For this review, take the finished solid that the model builds, in its own axes (mm). A direction names the side the tool comes from. Give positions to 0.01 mm unless a question says otherwise; leave off trailing zeros. Write each loop counter-clockwise with the first axis right and the second up, starting at its lowest first coordinate (ties: lowest second). Pieces come first, ordered by that corner, then holes. Notation, with made-up numbers: (-4.75, 9.5) -> (3.25, 9.5) arc R9 cw to (3.25, 24.5) -> close; hole circle Ø9 at (28, 30). An arc over 180 degrees is marked (long way). Write item = value, one per line.
```python
from build123d import *

# Parameters (mm, degrees)
CIRPATTERN1_COUNT         = 12
F_8_CLEARANCE_HOLE1_D     = 4.4958
F_8_CLEARANCE_HOLE1_DEPTH = 9.652
F_8_CLEARANCE_HOLE1_TIP   = 1.350674586


with BuildPart() as part:
    # Sketch1 → Revolve1 (revolve)
    with BuildSketch(Plane.XY, mode=Mode.PRIVATE) as revolve1_sk:
        Polygon((0, 0), (-30.6832, 0), (-30.6832, -7.8994), (-29.7942, -7.8994), (-29.7942, -12.319), (-26.1112, -12.319), (-26.1112, -6.223), (0, -6.223), align=None)
    revolve(revolve1_sk.sketch.rotate(Axis((0, -6.223, 0), (0, 1, 0)), 270), axis=Axis((0, -6.223, 0), (0, 1, 0)))

    # Sketch3 → D (0.246) Diameter Hole1 (revolve, cut)
    with BuildSketch(Plane(origin=(0, 0, -21.59), x_dir=(0, 0, 1), z_dir=(1, 0, 0))):
        Polygon((0, 0), (0, 14.577208746), (3.1242, 12.7), (3.1242, 0), align=None)
    d_0_246_diameter_hole1 = revolve(axis=Axis((0, 6.35, -21.59), (0, -1, 0)), mode=Mode.SUBTRACT)

    # CirPattern1: D (0.246) Diameter Hole1 ×12 about axis
    cirpattern1_axis = Axis((0, 0, 0), (0, 1, 0))
    for i in range(1, CIRPATTERN1_COUNT):
        add(d_0_246_diameter_hole1.rotate(cirpattern1_axis, i * 360 / CIRPATTERN1_COUNT), mode=Mode.SUBTRACT)

    # #8 Clearance Hole1
    with Locations(Plane.XZ.offset(6.223)):
        with Locations((0, 0)):
            Hole(F_8_CLEARANCE_HOLE1_D / 2, depth=F_8_CLEARANCE_HOLE1_DEPTH)
            with Locations((0, 0, -(F_8_CLEARANCE_HOLE1_DEPTH + F_8_CLEARANCE_HOLE1_TIP / 2))):  # 118° drill point
                Cone(0, F_8_CLEARANCE_HOLE1_D / 2, F_8_CLEARANCE_HOLE1_TIP, mode=Mode.SUBTRACT)


solid = part.part
```
(1) Take a section at C-C (z = -10.5). Write out the cut boundary in (x, y), plus the area to 3 significant figures.
Answers below:
outline = (-28.83, -7.9) -> (-27.88, -7.9) -> (-27.88, -12.32) -> (-23.91, -12.32) -> (-23.91, -6.22) -> (-21.81, -6.22) -> (-21.81, 0) -> (-28.83, 0) -> close; (-15.59, -6.22) -> (15.59, -6.22) -> (15.59, 0) -> (-15.59, 0) -> close; (21.81, -6.22) -> (23.91, -6.22) -> (23.91, -12.32) -> (27.88, -12.32) -> (27.88, -7.9) -> (28.83, -7.9) -> (28.83, 0) -> (21.81, 0) -> close
area = 333 mm^2
(2) Take a section at D-D (z = -20). Write out the cut boundary in (x, y).
Answers below:
outline = (-23.27, -7.9) -> (-22.08, -7.9) -> (-22.08, -12.32) -> (-16.79, -12.32) -> (-16.79, -6.22) -> (-13.63, -6.22) -> (-13.63, 0) -> (-23.27, 0) -> close; (-7.96, -6.22) -> (-2.69, -6.22) -> (-2.69, 0) -> (-7.96, 0) -> close; (2.69, -6.22) -> (7.96, -6.22) -> (7.96, 0) -> (2.69, 0) -> close; (13.63, -6.22) -> (16.79, -6.22) -> (16.79, -12.32) -> (22.08, -12.32) -> (22.08, -7.9) -> (23.27, -7.9) -> (23.27, 0) -> (13.63, 0) -> close
(3) For pin 1 (5 mm diameter, centred on y = -5, z = 14.5, fed in from -X); pin 2 (4 mm diameter, centred on x = 7, z = -16.5, fed in from -Y); pin 3 (5 mm diameter, centred on y = -10, z = 11, fed in from -X); pin 4 (3.5 mm diameter, centred on x = 10.8, z = 18.7, fed in from -Y), all flat-tipped, find the tip position at first contact; note any pin that passes through.
Answers below:
pin_1 = -28.24
pin_2 = -6.22
pin_3 = -29.13
pin_4 = through
(4) To check wall thickness, follow probe 1 along X at (y, z) = (-6, 2); probe 2 along X at (y, z) = (-3, -20); probe 3 along Z at (x, y) = (10, -1). State the ranges of each line that lie inside material, in increasing order.
Answers below:
probe_1 = -30.62 to -23.99, -19.19 to -1.03, 1.03 to 19.19, 23.99 to 30.62
probe_2 = -23.27 to -13.63, -7.96 to -2.69, 2.69 to 7.96, 13.63 to 23.27
probe_3 = -29.01 to -21.72, -15.68 to 15.68, 21.72 to 29.01
(5) The part is to be moulded in two halves that separate along X. For faces 3 (the face through (26.3, -12.319, 0.1)), 4 (the face through (-29.54, -10.14, 3.88)), 5 (the face through (8.316, -3.068, 16.796)), say which applies: released by +X, released by -X, zero draft, split by the parting line, or undercut.
Answers below:
face_3 = zero draft
face_4 = split by the parting line
face_5 = undercut
(6) Take a section at B-B (y = -4). Count the separate pieces of the cut face and the enclosed holes in it, plus the area to 3 significant figures.
Answers below:
separate_pieces = 1
enclosed_holes = 13
area = 2,570 mm^2
(7) Take a section at A-A (x = 0). Write out the cut boundary in (y, z).
Answers below:
outline = (-12.32, -29.79) -> (-7.9, -29.79) -> (-7.9, -30.68) -> (0, -30.68) -> (0, -24.71) -> (-6.22, -24.71) -> (-6.22, -26.11) -> (-12.32, -26.11) -> close; (-12.32, 26.11) -> (-6.22, 26.11) -> (-6.22, 24.71) -> (0, 24.71) -> (0, 30.68) -> (-7.9, 30.68) -> (-7.9, 29.79) -> (-12.32, 29.79) -> close; (-6.22, -18.47) -> (0, -18.47) -> (0, -2.25) -> (-6.22, -2.25) -> close; (-6.22, 2.25) -> (0, 2.25) -> (0, 18.47) -> (-6.22, 18.47) -> close
(8) Tool access review of faces 1 (the face through (-18.704, -3.068, -1.197)), 2 (the face through (-30, -7.899, 5)): name each direction out of +Z, -Z, +X, -X, +Y, -Y from which nothing blocks a thin tool from reaching the whole face with its end or side.
Answers below:
face_1 = +Y, -Y
face_2 = -Y
